Autodesk Inventor part; units mm, degrees
ref_plane "YZ Plane" through (0, 0, 0) normal (1, 0, 0) x (0, 1, 0)
ref_plane "XZ Plane" through (0, 0, 0) normal (0, 1, 0) x (-1, 0, 0)
ref_plane "XY Plane" through (0, 0, 0) normal (0, 0, 1) x (1, 0, 0)
sketch "Sketch1" plane through (0, 0, 0) normal (0, 1, 0) x (-1, 0, 0)
  circle A0 centre (0, 0) radius 12.7
  circle A1 centre (0, 0) radius 9.652
  circle A2 centre (0, 0) radius 38.1
  dimension "d0" = 25.4
  dimension "d1" = 19.304
  dimension "d2" = 76.2
extrude "Extrusion1" add sketch "Sketch1" along normal blind 6.35
sketch "Sketch2" plane through (0, 6.35, 0) normal (0, 1, 0) x (1, 0, 0)
  circle A0 centre (0, 0) radius 38.1
extrude "Extrusion2" add sketch "Sketch2" along normal blind 2.54
sketch "Sketch3" plane through (0, 0, 0) normal (0, -1, 0) x (1, 0, 0)
  circle A0 centre (0, 0) radius 38.1
extrude "Extrusion3" cut sketch "Sketch3" against normal blind 2.54
sketch "Sketch4" plane through (0, 2.54, 0) normal (0, -1, 0) x (1, 0, 0)
  circle A0 centre (0, 0) radius 19.05
  circle A1 centre (0, 0) radius 12.7
  circle A2 centre (0, 0) radius 9.652
  dimension "d9" = 38.1
extrude "Extrusion4" add sketch "Sketch4" along normal blind 6.35
sketch "Sketch5" plane through (0, 2.54, 0) normal (0, -1, 0) x (1, 0, 0)
  circle A0 centre (0, 0) radius 38.1
  line L0 (38.1, 0) -> (19.05, 0)
  circle A1 centre (0, 0) radius 19.05
  line L1 (0, 18.9941) -> (0, 38.0123)
  line L2 (-19.05, 0) -> (-38.1, 0)
  line L3 (0, -19.05) -> (0, -38.1)
  circle A2 centre (0, 28.5032) radius 1.5875
  circle A3 centre (28.575, 0) radius 1.5875
  circle A4 centre (0, -28.575) radius 1.5875
  circle A5 centre (-28.575, 0) radius 1.5875
  dimension "d12" = 3.175
  dimension "d13" = 3.175
  dimension "d14" = 3.175
  dimension "d15" = 3.175
extrude "Extrusion5" cut sketch "Sketch5" against normal blind 6.35 contours A2 L1 | L1 A2 | A3 L0 | L0 A3 | A5 L2 | L2 A5 | A4 L3 | L3 A4
properties part number "CrankAttachment_SBail"
Can you work these out from the model? Positions are in its coordinate system, mm. A direction names the side the tool comes from. Round coordinates to 2 decimals unless told otherwise and drop trailing zeros. Loops run counter-clockwise (first coordinate to the right, second up) from the corner with the lowest first, then second, coordinate; pieces in that order, holes last. Notation, with made-up numbers: (8.5, 46.5) - (16.5, 46.5) arc R12 ccw to (16.5, 64.5) - close; hole circle Ø7 at (-20.5, 58.25). An arc over 180 degrees is marked (long way). Use CSV: the item, a comma, the result in double quotes. Start each with the question number.
1) If we section it at C-C on y = -2: Write out the boundary of the cut face in (x, z), plus the area to 3 significant figures.
2) If we section it at B-B on x = 0: Write out the boundary of the cut face in (y, z).
3) For pin 1 Ø4 at (x, z) = (-28.575, 0) entering from +Y; pin 2 Ø1.5 at (x, y) = (-22, 1) entering from +Z; pin 3 Ø3.5 at (x, z) = (0, -28.575) entering from -Y; pin 4 Ø1 at (y, z) = (6, -11) entering from +X, each with a flat end and sliding along its axis, tell me the tip position at first contact or that it passes through.
4) If we section it at A-A on z = 0: Write out the boundary of the cut face in (x, y), plus the area to 3 significant figures.
5) We'd pull the mould along X, two halves only. Please class faces 1 (the flat face through (12.4, -3.81, -4)), 2 (the flat face through (2.8, 6.35, -9.5)), 3 (the cylindrical face through (-27.06, 5.67, 0.48)), 4 (the cylindrical face through (-15.12, -0.59, 11.59)): released by +X, released by -X, zero draft, split by the parting line, or undercut.
6) If we section it at D-D on x = -29: Write out the boundary of the cut face in (y, z), plus the area to 3 significant figures.
7) For faces 5 (the cylindrical face through (-0.207, 5.671, 30.077)), 6 (the flat face through (7.9, 2.54, 17.5)), which set-ups out of +Z, -Z, +X, -X, +Y, -Y let a thin tool reach every point of the face, with its end or its side?
8) Please list where these lines run through material, in increasing order: probe 1 along X at (y, z) = (5, 0); probe 2 along Z at (x, y) = (0, -0.5); probe 3 along Z at (x, y) = (0, 5.5). Write a range as [from, to].
Geometry results:
1,outline,"circle Ø38.1 at (0, 0); circle Ø19.3 at (0, 0); hole circle Ø25.4 at (0, 0)"
1,area,"926 mm2"
2,outline,"(-3.81, -19.05) - (2.54, -19.05) - (2.54, -26.99) - (8.89, -26.99) - (8.89, 26.92) - (2.54, 26.92) - (2.54, 19.05) - (-3.81, 19.05) - (-3.81, 12.7) - (6.35, 12.7) - (6.35, 9.65) - (-3.81, 9.65) - (-3.81, -9.65) - (6.35, -9.65) - (6.35, -12.7) - (-3.81, -12.7) - close; (2.54, -38.1) - (8.89, -38.1) - (8.89, -30.16) - (2.54, -30.16) - close; (2.54, 30.09) - (8.89, 30.09) - (8.89, 38.1) - (2.54, 38.1) - close"
3,pin 1,"stops at y = 8.89"
3,pin 2,"passes through"
3,pin 3,"stops at y = 2.54"
3,pin 4,"stops at x = 36.62"
4,outline,"(-38.1, 2.54) - (-30.16, 2.54) - (-30.16, 8.89) - (-38.1, 8.89) - close; (-26.99, 2.54) - (-19.05, 2.54) - (-19.05, -3.81) - (-12.7, -3.81) - (-12.7, 6.35) - (-9.65, 6.35) - (-9.65, -3.81) - (9.65, -3.81) - (9.65, 6.35) - (12.7, 6.35) - (12.7, -3.81) - (19.05, -3.81) - (19.05, 2.54) - (26.99, 2.54) - (26.99, 8.89) - (-26.99, 8.89) - close; (30.16, 2.54) - (38.1, 2.54) - (38.1, 8.89) - (30.16, 8.89) - close"
4,area,"624 mm2"
5,face 1,"zero draft"
5,face 2,"undercut"
5,face 3,"undercut"
5,face 4,"split by the parting line"
6,outline,"(2.54, -24.71) - (8.89, -24.71) - (8.89, -1.53) - (2.54, -1.53) - close; (2.54, 1.53) - (8.89, 1.53) - (8.89, 24.71) - (2.54, 24.71) - close"
6,area,"294 mm2"
7,face 5,"+Y, -Y"
7,face 6,"-Y"
8,probe 1,"x = [-38.1, -30.16], [-26.99, -12.7], [-9.65, 9.65], [12.7, 26.99], [30.16, 38.1]"
8,probe 2,"z = [-19.05, -12.7], [-9.65, 9.65], [12.7, 19.05]"
8,probe 3,"z = [-38.1, -30.16], [-26.99, -12.7], [-9.65, 9.65], [12.7, 26.92], [30.09, 38.1]"
